Job drawing, mm, ordinate dimensions from the low corner. One solid piece. A direction names the side the tool comes from. Give positions to 0.01 mm unless a question says otherwise; leave off trailing zeros. Write each loop counter-clockwise with the first axis right and the second up, starting at its lowest first coordinate (ties: lowest second). Pieces come first, ordered by that corner, then holes. Notation, with made-up numbers: (16.25, 66) -> (49.25, 66) arc R16 cw to (49.25, 70) -> close; hole circle Ø9 at (74, -33). An arc over 180 degrees is marked (long way). One line per question, with ' | ' between items. Start each with the question number.
(1) Band-saw the part on A-A, the plane y = 123.75. Give the cut face in (x, z), and give its area (3 significant figures).
(2) Pin check, flat tips, straight feed: P1, Ø8, axis at x = 11, y = 123.75, coming from the -Z side; P2, Ø3.5, axis at x = 154, y = 123.75, coming from the -Z side (1 decimal); P3, Ø6.5, axis at y = 49, z = 4.5, coming from the +X side; P4, Ø4, axis at y = 60, z = 3, coming from the -X side. Stop position of each tip, or through.
(3) Tool access for the marked faces 1, 2, 3, 4 and 5: list every direction of +Z, -Z, +X, -X, +Y, -Y with a clear straight run to the whole face (end or side of a thin tool).
(4) Band-saw the part on B-B, the plane x = 11. Give the cut face in (y, z), and give its area (3 significant figures).
(5) Band-saw the part on D-D, the plane x = 100.5. Give the cut face in (y, z).
(6) Band-saw the part on C-C, the plane y = 109.5. Give the cut face in (x, z).
(7) Drill centre lines: probe 1 along X at (y, z) = (123.75, 9.6); probe 2 along Y at (x, z) = (11, 9.75); probe 3 along X at (y, z) = (84.5, 5). Where is each one in solid material? Low to high. Write a range as from..to.
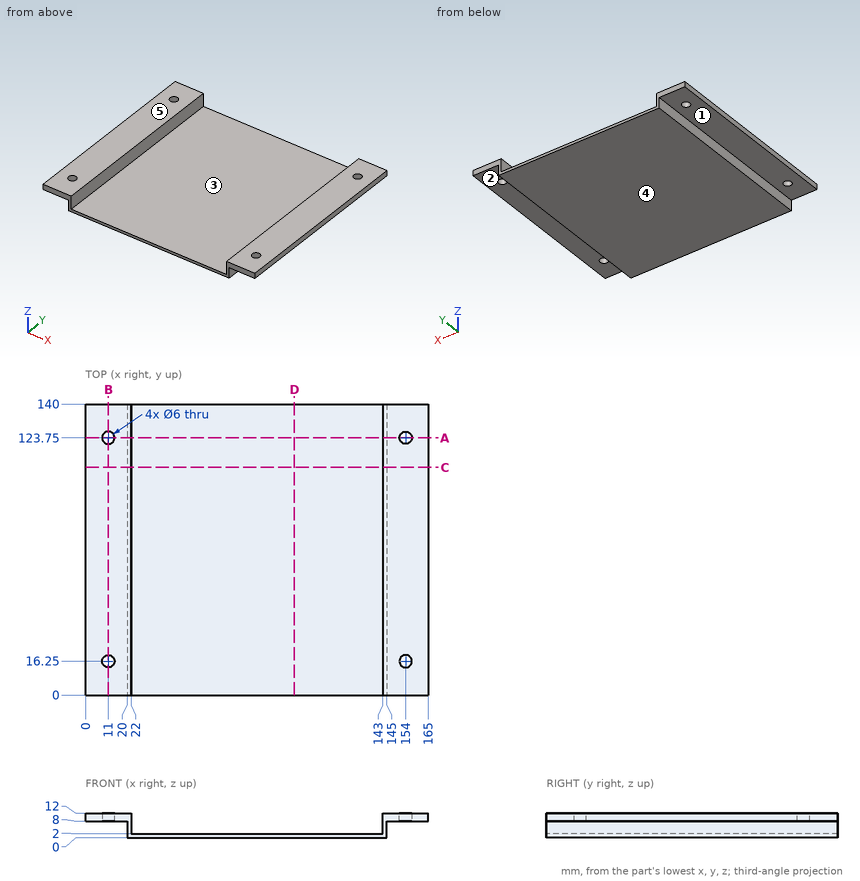
Results:
1) outline: (0, 8) -> (8, 8) -> (8, 12) -> (0, 12) -> close; (14, 8) -> (20, 8) -> (20, 0) -> (145, 0) -> (145, 8) -> (151, 8) -> (151, 12) -> (143, 12) -> (143, 2) -> (22, 2) -> (22, 12) -> (14, 12) -> close; (157, 8) -> (165, 8) -> (165, 12) -> (157, 12) -> close | area: 402 mm²
2) P1: stops at z = 8 | P2: passes through | P3: stops at x = 145 | P4: stops at x = 20
3) face 1: -Z, -X, +Y, -Y | face 2: -Z, +X, +Y, -Y | face 3: +Z, +Y, -Y | face 4: -Z, +X, -X, +Y, -Y | face 5: +Z, +X, -X, +Y, -Y
4) outline: (0, 8) -> (13.25, 8) -> (13.25, 12) -> (0, 12) -> close; (19.25, 8) -> (120.75, 8) -> (120.75, 12) -> (19.25, 12) -> close; (126.75, 8) -> (140, 8) -> (140, 12) -> (126.75, 12) -> close | area: 512 mm²
5) outline: (0, 0) -> (140, 0) -> (140, 2) -> (0, 2) -> close
6) outline: (0, 8) -> (20, 8) -> (20, 0) -> (145, 0) -> (145, 8) -> (165, 8) -> (165, 12) -> (143, 12) -> (143, 2) -> (22, 2) -> (22, 12) -> (0, 12) -> close
7) probe 1: x = 0..8, 14..22, 143..151, 157..165 | probe 2: y = 0..13.25, 19.25..120.75, 126.75..140 | probe 3: x = 20..22, 143..145
